For this review, take the finished solid that the model builds, in its own axes (mm). A direction names the side the tool comes from. Coordinates: 2 decimals unless noted, no trailing zeros. Write each loop counter-clockwise with the first axis right and the second up, starting at its lowest first coordinate (ties: lowest second). Pieces come first, ordered by that corner, then holes.
1) We need section A-A on y = 14.08. Write out the cut boundary in (x, z) (3 decimals).
2) We need section C-C on z = 6. Write out the cut boundary in (x, y) (3 decimals).
3) Mouldability with a two-part tool opening along X and no side actions: class faces 4 (the face through (23.068, 15.097, 5.576)), 5 (the face through (77, 0, 3)), 6 (the face through (94.928, 12.985, 2.105)), 7 (the face through (56.669, 12.483, 2.105)) as pulls with the +X half, pulls with the -X half, needs draft (parallel to the pull), parting line crosses it, or undercut.
4) Insertion check: P1, Ø2, axis at x = 93.5, y = 14.08, coming from the -Z side; P2, Ø3, axis at x = 19.5, y = 13.5, coming from the +Z side; P3, Ø5.5, axis at x = 99.5, y = 21.7, coming from the -Z side; P4, Ø1, axis at x = 43, y = 26.5, coming from the +Z side. Each pin has a flat end and moves straight along its axis. Give the tip position at first contact, or say it passes through.
5) To check wall thickness, follow line 1 along X through (y, z) = (21.5, 0.5); line 2 along Y through (x, z) = (99.5, 5.55); line 3 along Y through (x, z) = (57.5, 5.75) (3 decimals). State the ranges of each line that lie inside material, in increasing order.
6) For faces 1 (the face through (74, 16, 0)), 2 (the face through (58.9, 12.7, 4.27)), 3 (the face through (98, 20, 3.81)), list the 3-axis set-ups (+Z, -Z, +X, -X, +Y, -Y) from which the entire face can be reached by the end or side of a thin tool; tool diameter is ignored.
7) We need section D-D on y = 27. Write out the cut boundary in (x, z).
8) We need section B-B on x = 93.5. Write out the cut boundary in (y, z) (3 decimals), then the cut area to 3 significant figures.
Autodesk Inventor part; units mm, degrees
ref_plane "Work Plane2" through (0, 0, 8.08) normal (0, 0, 1) x (1, 0, 0)
ref_plane "YZ Plane" through (0, 0, 0) normal (1, 0, 0) x (0, 1, 0)
ref_plane "XZ Plane" through (0, 0, 0) normal (0, 1, 0) x (-1, 0, 0)
sketch "Sketch1" plane through (0, 0, 0) normal (0, 0, 1) x (1, 0, 0)
  line L0 (0, 0) -> (151, 0)
  line L1 (151, 0) -> (151, 30.623)
  line L2 (151, 30.623) -> (0, 30.623)
  line L3 (0, 30.623) -> (0, 0)
  dimension "d0" = 151
  dimension "d1" = 30.623
extrude "Extrusion1" add sketch "Sketch1" along normal blind 3
ref_plane "Work Plane2" through (0, 0, 8.08) normal (0, 0, 1) x (1, 0, 0)
sketch "Sketch2" plane through (0, 0, 8.08) normal (0, 0, 1) x (1, 0, 0)
  line L0 (151, 0) -> (151, 30.623) construction
  line L1 (151, 30.623) -> (0, 30.623) construction
  line L2 (0, 30.623) -> (0, 0)
  line L3 (0, 0) -> (151, 0) construction
  line L4 (45.5, 30.623) -> (105.5, 30.623)
  line L5 (105.5, 30.623) -> (105.5, 0)
  line L6 (105.5, 0) -> (45.5, 0)
  line L7 (45.5, 0) -> (45.5, 30.623)
  line L8 (45.5, 15.3115) -> (0, 15.3115) construction
  line L9 (105.5, 15.3115) -> (151, 15.3115) construction
  dimension "d6" = 60
loft "Loft1" add profiles "Sketch2" section 1 edges at (151, 15.3115, 3) (75.5, 30.623, 3) (0, 15.3115, 3) (75.5, 0, 3)
sketch "Sketch7" plane through (0, 0, 0) normal (0, 0, -1) x (-1, 0, 0)
  circle A0 centre (-93.5, 14.08) radius 1.8
  circle A1 centre (-57.5, 14.08) radius 1.8
  line L0 (0, 0) -> (-151, 0)
  line L1 (-151, 0) -> (-151, 30.623)
  line L2 (0, 30.623) -> (0, 0)
  dimension "d25" = 14.08
  dimension "d26" = 14.08
  dimension "d27" = 57.5
  dimension "d28" = 3.6
  dimension "d29" = 57.5
  dimension "d30" = 3.6
extrude "Extrusion4" cut sketch "Sketch7" along normal mid plane 225.25
sketch "Sketch8" plane through (45.5, 30.623, 8.08) normal (0, 0, 1) x (1, 0, 0)
  circle A0 centre (48, -16.543) radius 1.8
  circle A1 centre (12, -16.543) radius 1.8
  line L0 (60, 0) -> (60, -30.623)
  line L1 (0, 0) -> (60, 0)
  line L2 (0, -30.623) -> (0, 0)
  line L3 (60, -30.623) -> (0, -30.623)
  circle A2 centre (12, -16.543) radius 3.175
  circle A3 centre (48, -16.543) radius 3.175
  point P0 (-45.5, -30.623)
  dimension "d33" = 6.35
  dimension "d34" = 6.35
extrude "Extrusion5" cut sketch "Sketch8" against normal blind 3.81 contours A0 | A1 | A2 | A3
sketch "Sketch9" plane through (0, 0, 0) normal (0, 0, -1) x (-1, 0, 0)
  circle A0 centre (-75.5, 21.7) radius 1.8
  circle A1 centre (-99.5, 21.7) radius 1.8
  circle A2 centre (-93.5, 14.08) radius 1.8
  circle A3 centre (-57.5, 14.08) radius 1.8
  line L0 (-151, 0) -> (-151, 30.623)
  line L1 (0, 0) -> (-151, 0)
  line L2 (0, 30.623) -> (0, 0)
  line L3 (-151, 30.623) -> (0, 30.623)
  line L4 (-75.5, 21.7) -> (-75.5, 0) construction
  line L5 (-75.5, 21.7) -> (-99.5, 21.7) construction
  dimension "d37" = 3.6
  dimension "d38" = 3.6
  dimension "d40" = 24
  dimension "d43" = 7.62
extrude "Extrusion6" cut sketch "Sketch9" along normal mid plane 73.66 contours A0 | A1
sketch "Sketch11" plane through (0, 0, 0) normal (0, 0, -1) x (-1, 0, 0)
  circle A0 centre (-99.5, 21.7) radius 1.8
  circle A1 centre (-75.5, 21.7) radius 1.8
  circle A2 centre (-93.5, 14.08) radius 1.8
  circle A3 centre (-57.5, 14.08) radius 1.8
  line L0 (-151, 0) -> (-151, 30.623)
  line L1 (0, 0) -> (-151, 0)
  line L2 (0, 30.623) -> (0, 0)
  line L3 (-151, 30.623) -> (0, 30.623)
  circle A4 centre (-75.5, 21.7) radius 3.175
  circle A5 centre (-99.5, 21.7) radius 3.175
  dimension "d44" = 6.35
  dimension "d45" = 6.35
extrude "Extrusion7" cut sketch "Sketch11" against normal blind 3.81 contours A0 | A1 | A4 | A5
properties part number "ZED_mount_V2_3DPrint"
Result:
1. outline: (0, 0) - (55.7, 0) - (55.7, 4.27) - (54.325, 4.27) - (54.325, 8.08) - (45.5, 8.08) - (0, 3) - close; (59.3, 0) - (91.7, 0) - (91.7, 4.27) - (90.325, 4.27) - (90.325, 8.08) - (60.675, 8.08) - (60.675, 4.27) - (59.3, 4.27) - close; (95.3, 0) - (151, 0) - (151, 3) - (105.5, 8.08) - (96.675, 8.08) - (96.675, 4.27) - (95.3, 4.27) - close
2. outline: (26.87, 0) - (124.13, 0) - (124.13, 30.623) - (26.87, 30.623) - close; hole circle Ø6.35 at (57.5, 14.08); hole circle Ø3.6 at (75.5, 21.7); hole circle Ø6.35 at (93.5, 14.08); hole circle Ø3.6 at (99.5, 21.7)
3. face 4: pulls with the -X half
3. face 5: needs draft
3. face 6: undercut
3. face 7: undercut
4. P1: passes through
4. P2: stops at z = 5.34
4. P3: stops at z = 3.81
4. P4: stops at z = 7.86
5. line 1: x = 0 to 72.33, 78.67 to 96.33, 102.67 to 151
5. line 2: y = 0 to 19.9, 23.5 to 30.62
5. line 3: y = 0 to 10.905, 17.255 to 30.623
6. face 1: -Z, +X, -X, +Y, -Y
6. face 2: +Z
6. face 3: -Z
7. outline: (0, 0) - (151, 0) - (151, 3) - (105.5, 8.08) - (45.5, 8.08) - (0, 3) - close
8. outline: (0, 0) - (12.28, 0) - (12.28, 4.27) - (10.905, 4.27) - (10.905, 8.08) - (0, 8.08) - close; (15.88, 0) - (30.623, 0) - (30.623, 8.08) - (17.255, 8.08) - (17.255, 4.27) - (15.88, 4.27) - close
8. area: 208 mm2
